from build123d import *

# Parameters (mm, degrees)
F0_R     = 21
F0_R_2   = 19
F1_DEPTH = 210
F3_DEPTH = 500
F5_DEPTH = 500


with BuildPart() as f1:
    # F0 (on Top) → F1 (new body)
    with BuildSketch(Plane.XY):
        Circle(F0_R)
        Circle(F0_R_2, mode=Mode.SUBTRACT)
    extrude(amount=F1_DEPTH)

    # F2 (on Front) → F3 (cut, symmetric)
    with BuildSketch(Plane.XZ):
        Polygon((-1.5875, 67), (-1.5875, 17), (0, 17), (1.5875, 17), (1.5875, 67), align=None)
    extrude(amount=F3_DEPTH, both=True, mode=Mode.SUBTRACT)

    # F4 (on Right) → F5 (cut, symmetric)
    with BuildSketch(Plane.YZ):
        Polygon((0, 17), (1.5875, 17), (1.5875, 67), (-1.5875, 67), (-1.5875, 17), align=None)
    extrude(amount=F5_DEPTH, both=True, mode=Mode.SUBTRACT)


solid = f1.part
Geometry check sheet. Reference: the model listing, model coordinates, mm. Coordinates: 2 decimals unless noted, no trailing zeros. Loops run counter-clockwise (first coordinate to the right, second up) from the corner with the lowest first, then second, coordinate; pieces in that order, holes last. Notation, with made-up numbers: (30, -30) - (78, -30) arc R11 cw to (78, -19) - close; hole circle Ø1 at (18.25, 16). An arc over 180 degrees is marked (long way). Use one line per item in the form item = value. Start each with the question number.
Item 1: Section check A-A, the plane x = 12.5. Enter the section's corners in (y, z), and give its area (3 significant figures).
Item 2: Mould release check, pull along X, two halves, no side actions. Record for faces 1 (the face through (20.03, 6.31, 103.53)), 2 (the face through (-16, -11, 0)), 3 (the face through (18.12, 5.71, 103.53)): +X half, -X half, draft (parallel to the pull), parting line (faces both ways), or undercut.
Item 3: Section check C-C, the plane z = 185.5. Enter the section's corners in (x, y), and give its area (3 significant figures).
Item 4: Section check B-B, the plane y = -4. Enter the section's corners in (x, z).
Item 5: Gauge pin test, flat ends, axial feed: pin 1 (6 mm diameter, centred on y = 7, z = 58.5, fed in from +X); pin 2 (2 mm diameter, centred on x = -10.5, z = 151, fed in from +Y); pin 3 (1 mm diameter, centred on y = -5, z = 65.5, fed in from -X). Record the tip position at first contact, or that the pin passes through.
Item 6: Thickness scan on probe 1 along X at (y, z) = (0, 89); probe 2 along Y at (x, z) = (1.5, 124). Record the ranges inside material, lowest first.
Computed:
q1.outline = (-16.87, 0) - (-14.31, 0) - (-14.31, 210) - (-16.87, 210) - close; (14.31, 0) - (16.87, 0) - (16.87, 210) - (14.31, 210) - close
q1.area = 1,080 mm2
q2.face_1 = parting line
q2.face_2 = draft
q2.face_3 = undercut
q3.outline = circle Ø42 at (0, 0); hole circle Ø38 at (0, 0)
q3.area = 251 mm2
q4.outline = (-20.62, 0) - (-18.57, 0) - (-18.57, 210) - (-20.62, 210) - close; (18.57, 0) - (20.62, 0) - (20.62, 210) - (18.57, 210) - close
q5.pin_1 = 20.62
q5.pin_2 = 18.73
q5.pin_3 = -20.51
q6.probe_1 = -21 to -19, 19 to 21
q6.probe_2 = -20.95 to -18.94, 18.94 to 20.95
